```python
from build123d import *

# Parameters (mm, degrees)
SKETCH1_R           = 8
BOSS_EXTRUDE1_DEPTH = 2.5
FILLET1_R           = 3
SKETCH2_W           = 25
SKETCH2_H           = 3
BOSS_EXTRUDE2_DEPTH = 12
FILLET2_R           = 2.5
FILLET3_R           = 3
SKETCH3_R           = 1.5
CUT_EXTRUDE1_DEPTH  = 44.462627624


with BuildPart() as part:
    # Sketch1 → Boss-Extrude1 (new body)
    with BuildSketch(Plane.XY):
        with BuildLine():
            Line((-28, -15), (-28, -0.5))
            ThreePointArc((-28, -0.5), (-23.460155108, 10.460155108), (-12.5, 15))
            Line((-12.5, 15), (12.5, 15))
            ThreePointArc((12.5, 15), (23.460155108, 10.460155108), (28, -0.5))
            Line((28, -0.5), (28, -15))
            Line((28, -15), (12.5, -15))
            Line((12.5, -15), (12.5, -19))
            Line((12.5, -19), (-12.5, -19))
            Line((-12.5, -19), (-12.5, -15))
            Line((-12.5, -15), (-28, -15))
        make_face()
        with Locations((12.5, -0.5)):
            Circle(SKETCH1_R, mode=Mode.SUBTRACT)
        with Locations((-12.5, -0.5)):
            Circle(SKETCH1_R, mode=Mode.SUBTRACT)
    extrude(amount=BOSS_EXTRUDE1_DEPTH)

    # Fillet1
    fillet1_edges = [part.edges().sort_by_distance(p)[0] for p in [
        (-28, -15, 1.25),
        (28, -15, 1.25),
    ]]
    fillet(fillet1_edges, radius=FILLET1_R)

    # Sketch2 → Boss-Extrude2 (add)
    with BuildSketch(Plane(origin=(0, 0, 0), x_dir=(-1, 0, 0), z_dir=(0, 0, -1))):
        with Locations((0, -17.5)):
            Rectangle(SKETCH2_W, SKETCH2_H)
    extrude(amount=BOSS_EXTRUDE2_DEPTH)

    # Fillet2
    fillet2_edges = [part.edges().sort_by_distance(p)[0] for p in [
        (12.5, -17.5, -12),
        (-12.5, -17.5, -12),
    ]]
    fillet(fillet2_edges, radius=FILLET2_R)

    # Fillet3
    fillet3_edges = [part.edges().sort_by_distance(p)[0] for p in [
        (0, -19, 2.5),
    ]]
    fillet(fillet3_edges, radius=FILLET3_R)

    # Sketch3 → Cut-Extrude1 (cut, through all)
    with BuildSketch(Plane(origin=(0, -16, 0), x_dir=(1, 0, 0), z_dir=(0, 1, 0))):
        with Locations(Location((0, 7, 0), (0, 0, 270))):
            Circle(SKETCH3_R)
    extrude(amount=-CUT_EXTRUDE1_DEPTH, mode=Mode.SUBTRACT)


solid = part.part
```
Geometry: final body of the model. Coordinates: model frame, mm. A direction names the side the tool comes from. Round coordinates to 2 decimals unless told otherwise and drop trailing zeros. Loops run counter-clockwise (first coordinate to the right, second up) from the corner with the lowest first, then second, coordinate; pieces in that order, holes last. Notation, with made-up numbers: (6, -6.75) -> (14, -6.75) arc R16 cw to (14, 14.25) -> close; hole circle Ø4 at (-20.75, 35). An arc over 180 degrees is marked (long way). Use one line per item in the form item = value. Start each with the question number.
1) Section C-C on y = 5. Output: boundary loops of the cut face in (x, z).
2) Section A-A on x = 0. Output: boundary loops of the cut face in (y, z).
3) Access query for faces 1 (the flat face through (0, 0, 0)), 2 (the flat face through (-19, -15, 1)), 3 (the cylindrical face through (23.34, 10.58, 1.23)), 4 (the flat face through (12.5, -17, -3)). Directions: +Z, -Z, +X, -X, +Y, -Y. A direction counts if a zero-diameter tool reaches every point of the face in a straight line with its end or side. Return the directions, or none.
4) Line query: L1, parallel to X at y = -3, z = 1.5; L2, parallel to Y at x = -8, z = -3; L3, parallel to Z at x = -24, y = -1.5. Output: solid intervals per line, ascending.
5) First-contact query: P1, Ø3, axis at x = 18.5, z = 2, coming from the -Y side; P2, Ø9.5, axis at x = 12.5, y = -0.5, coming from the -Z side; P3, Ø4.5, axis at y = -16.5, z = -3, coming from the -X side; P4, Ø2, axis at y = -18, z = -5.5, coming from the +X side. Flat tips, straight axial feed; report the tip coordinate or a pass-through.
6) Section D-D on x = -15. Output: boundary loops of the cut face in (y, z), then the cut area to 3 significant figures.
7) Section B-B on z = -7. Output: boundary loops of the cut face in (x, y).
8) Draft query along X for faces 5 (the cylindrical face through (10.77, -8.31, 1.23)), 6 (the cylindrical face through (-23.58, 10.34, 1.23)), 7 (the flat face through (19, -15, 1)). Return one class per face: released by +X, released by -X, zero draft, split by the parting line, or undercut.
Response:
q1.outline = (-26.99, 0) -> (-18.31, 0) -> (-18.31, 2.5) -> (-26.99, 2.5) -> close; (-6.69, 0) -> (6.69, 0) -> (6.69, 2.5) -> (-6.69, 2.5) -> close; (18.31, 0) -> (26.99, 0) -> (26.99, 2.5) -> (18.31, 2.5) -> close
q2.outline = (-19, -12) -> (-16, -12) -> (-16, -8.5) -> (-19, -8.5) -> close; (-19, -5.5) -> (-16, -5.5) -> (-16, 0) -> (15, 0) -> (15, 2.5) -> (-16, 2.5) arc R3 ccw to (-19, -0.5) -> close
q3.face_1 = -Z, +X, -X, +Y
q3.face_2 = +Z, -Z, -X, -Y
q3.face_3 = +Z, -Z, +X, +Y
q3.face_4 = +Z, -Z, +X, -Y
q4.L1 = -28 to -20.1, -4.9 to 4.9, 20.1 to 28
q4.L2 = -19 to -16
q4.L3 = 0 to 2.5
q5.P1 = -15
q5.P2 = through
q5.P3 = -12.5
q5.P4 = 12.5
q6.outline = (-15, 0) -> (-8.1, 0) -> (-8.1, 2.5) -> (-15, 2.5) -> close; (7.1, 0) -> (14.8, 0) -> (14.8, 2.5) -> (7.1, 2.5) -> close
q6.area = 36.5 mm^2
q7.outline = (-12.5, -19) -> (-1.5, -19) -> (-1.5, -16) -> (-12.5, -16) -> close; (1.5, -19) -> (12.5, -19) -> (12.5, -16) -> (1.5, -16) -> close
q8.face_5 = undercut
q8.face_6 = released by -X
q8.face_7 = zero draft
